For this review, take the finished solid that the model builds, in its own axes (mm). A direction names the side the tool comes from. Give positions to 0.01 mm unless a question says otherwise; leave off trailing zeros. Loops run counter-clockwise (first coordinate to the right, second up) from the corner with the lowest first, then second, coordinate; pieces in that order, holes last. Notation, with made-up numbers: (28, -9.5) - (85, -9.5) arc R13 cw to (85, -0.5) - close; hole circle Ø7 at (88.25, -26). An arc over 180 degrees is marked (long way). Answer in a Markdown table with one row per item.
```python
from build123d import *

# Parameters (mm, degrees)
SKETCH1_R                     = 44.45
SKETCH1_R_2                   = 3.25
BOSS_EXTRUDE1_DEPTH           = 3.175
BOSS_EXTRUDE2_DEPTH           = 67.31
CBORE_FOR_M6_SHCS2_AT_2_COUNT = 2
CBORE_FOR_M6_SHCS2_AT_2_PITCH = 111.76
CBORE_FOR_M6_SHCS2_AT_3_COUNT = 2
CBORE_FOR_M6_SHCS2_AT_3_PITCH = 158.052507731
CBORE_FOR_M6_SHCS2_AT_4_COUNT = 2
CBORE_FOR_M6_SHCS2_AT_4_PITCH = 111.76


with BuildPart() as part:
    # Sketch1 → Boss-Extrude1 (new body)
    with BuildSketch(Plane(origin=(0, 0, 0), x_dir=(1, 0, 0), z_dir=(0, 1, 0))):
        with BuildLine():
            Line((-57.15, 63.5), (57.15, 63.5))
            ThreePointArc((57.15, 63.5), (61.640128061, 61.640128061), (63.5, 57.15))
            Line((63.5, 57.15), (63.5, -57.15))
            ThreePointArc((63.5, -57.15), (61.640128061, -61.640128061), (57.15, -63.5))
            Line((57.15, -63.5), (-57.15, -63.5))
            ThreePointArc((-57.15, -63.5), (-61.640128061, -61.640128061), (-63.5, -57.15))
            Line((-63.5, -57.15), (-63.5, 57.15))
            ThreePointArc((-63.5, 57.15), (-61.640128061, 61.640128061), (-57.15, 63.5))
        make_face()
        Circle(SKETCH1_R, mode=Mode.SUBTRACT)
        with Locations((-57.15, 53.975)):
            Circle(SKETCH1_R_2, mode=Mode.SUBTRACT)
        with Locations((57.15, 53.975)):
            Circle(SKETCH1_R_2, mode=Mode.SUBTRACT)
        with Locations((57.15, -53.975)):
            Circle(SKETCH1_R_2, mode=Mode.SUBTRACT)
        with Locations((-57.15, -53.975)):
            Circle(SKETCH1_R_2, mode=Mode.SUBTRACT)
    extrude(amount=BOSS_EXTRUDE1_DEPTH)

    # Sketch3 → Boss-Extrude2 (add)
    with BuildSketch(Plane(origin=(0, 3.175, 0), x_dir=(1, 0, 0), z_dir=(0, 1, 0))):
        with BuildLine():
            Line((-57.15, -63.5), (57.15, -63.5))
            ThreePointArc((57.15, -63.5), (61.640128061, -61.640128061), (63.5, -57.15))
            Line((63.5, -57.15), (63.5, 57.15))
            ThreePointArc((63.5, 57.15), (61.640128061, 61.640128061), (57.15, 63.5))
            Line((57.15, 63.5), (-57.15, 63.5))
            ThreePointArc((-57.15, 63.5), (-61.640128061, 61.640128061), (-63.5, 57.15))
            Line((-63.5, 57.15), (-63.5, -57.15))
            ThreePointArc((-63.5, -57.15), (-61.640128061, -61.640128061), (-57.15, -63.5))
        make_face()
        with BuildLine():
            Line((-54.700256121, 45.358975516), (-45.358975516, 54.700256121))
            ThreePointArc((-45.358975516, 54.700256121), (-41.238798986, 57.453270063), (-36.378719395, 58.42))
            Line((-36.378719395, 58.42), (36.378719395, 58.42))
            ThreePointArc((36.378719395, 58.42), (41.238798986, 57.453270063), (45.358975516, 54.700256121))
            Line((45.358975516, 54.700256121), (54.700256121, 45.358975516))
            ThreePointArc((54.700256121, 45.358975516), (57.453270063, 41.238798986), (58.42, 36.378719395))
            Line((58.42, 36.378719395), (58.42, -36.378719395))
            ThreePointArc((58.42, -36.378719395), (57.453270063, -41.238798986), (54.700256121, -45.358975516))
            Line((54.700256121, -45.358975516), (45.358975516, -54.700256121))
            ThreePointArc((45.358975516, -54.700256121), (41.238798986, -57.453270063), (36.378719395, -58.42))
            Line((36.378719395, -58.42), (-36.378719395, -58.42))
            ThreePointArc((-36.378719395, -58.42), (-41.238798986, -57.453270063), (-45.358975516, -54.700256121))
            Line((-45.358975516, -54.700256121), (-54.700256121, -45.358975516))
            ThreePointArc((-54.700256121, -45.358975516), (-57.453270063, -41.238798986), (-58.42, -36.378719395))
            Line((-58.42, -36.378719395), (-58.42, 36.378719395))
            ThreePointArc((-58.42, 36.378719395), (-57.453270063, 41.238798986), (-54.700256121, 45.358975516))
        make_face(mode=Mode.SUBTRACT)
    extrude(amount=BOSS_EXTRUDE2_DEPTH)

    # Sketch9 → CBORE for M6 SHCS2 (revolve, cut)
    with BuildSketch(Plane(origin=(55.88, 0, -55.88), x_dir=(0, 0, -1), z_dir=(1, 0, 0))):
        Polygon((0, 0), (0, 70.485), (3.5, 70.485), (3.5, 31.4), (5.5, 31.4), (5.5, 0.025), (5.525, 0), align=None)
    cbore_for_m6_shcs2 = revolve(axis=Axis((55.88, -6.35, -55.88), (0, 1, 0)), mode=Mode.SUBTRACT)

    # CBORE for M6 SHCS2 at 2: CBORE for M6 SHCS2 ×2
    with Locations(*[(-i * CBORE_FOR_M6_SHCS2_AT_2_PITCH, 0, 0) for i in range(1, CBORE_FOR_M6_SHCS2_AT_2_COUNT)]):
        add(cbore_for_m6_shcs2, mode=Mode.SUBTRACT)

    # CBORE for M6 SHCS2 at 3: CBORE for M6 SHCS2 ×2
    with Locations(*[Vector(-0.707106781, 0, 0.707106781) * (i * CBORE_FOR_M6_SHCS2_AT_3_PITCH) for i in range(1, CBORE_FOR_M6_SHCS2_AT_3_COUNT)]):
        add(cbore_for_m6_shcs2, mode=Mode.SUBTRACT)

    # CBORE for M6 SHCS2 at 4: CBORE for M6 SHCS2 ×2
    with Locations(*[(0, 0, i * CBORE_FOR_M6_SHCS2_AT_4_PITCH) for i in range(1, CBORE_FOR_M6_SHCS2_AT_4_COUNT)]):
        add(cbore_for_m6_shcs2, mode=Mode.SUBTRACT)


solid = part.part
```
1. Clearance check with flat-ended pins moving along their axes: pin 1 (10 mm diameter, centred on x = -22.5, z = 27.5, fed in from +Y); pin 2 (12 mm diameter, centred on x = 55, z = -56.5, fed in from -Y); pin 3 (6 mm diameter, centred on x = -38, z = -22.5, fed in from +Y) (3 decimals). State where each tip first meets the part, or that it passes through.
Values:
| item | result |
|---|---|
| pin 1 | passes through |
| pin 2 | stops at y = 0 |
| pin 3 | stops at y = 3.175 |
2. We need section C-C, the plane z = 0. Give the boundary of the cut face in (x, y) (3 decimals).
Values:
| item | result |
|---|---|
| outline | (-63.5, 0) - (-44.45, 0) - (-44.45, 3.175) - (-58.42, 3.175) - (-58.42, 70.485) - (-63.5, 70.485) - close; (44.45, 0) - (63.5, 0) - (63.5, 70.485) - (58.42, 70.485) - (58.42, 3.175) - (44.45, 3.175) - close |
3. We need section B-B, the plane x = 0. Give the boundary of the cut face in (y, z) (3 decimals), and give its area (3 significant figures).
Values:
| item | result |
|---|---|
| outline | (0, -63.5) - (70.485, -63.5) - (70.485, -58.42) - (3.175, -58.42) - (3.175, -44.45) - (0, -44.45) - close; (0, 44.45) - (3.175, 44.45) - (3.175, 58.42) - (70.485, 58.42) - (70.485, 63.5) - (0, 63.5) - close |
| area | 805 mm^2 |
4. Mouldability with a two-part tool opening along X and no side actions: class faces 1 (the face through (57, 31.4, 59.5)), 2 (the face through (1, 35, -63.5)), 3 (the face through (-63.5, 35, -1)) as released by +X, released by -X, zero draft, split by the parting line, or undercut.
Values:
| item | result |
|---|---|
| face 1 | undercut |
| face 2 | zero draft |
| face 3 | released by -X |
5. For faces 4 (the face through (-50.1, 36.36, -49.96)), 5 (the face through (56, 31.4, -52)), 6 (the face through (-56.034, 50.669, -52.383)), list the 3-axis set-ups (+Z, -Z, +X, -X, +Y, -Y) from which the entire face can be reached by the end or side of a thin tool; tool diameter is ignored.
Values:
| item | result |
|---|---|
| face 4 | +Y |
| face 5 | -Y |
| face 6 | +Y, -Y |
6. We need section A-A, the plane y = 21. Give the boundary of the cut face in (x, z), and give its area (3 significant figures).
Values:
| item | result |
|---|---|
| outline | (-63.5, -57.15) arc R6.35 ccw to (-57.15, -63.5) - (57.15, -63.5) arc R6.35 ccw to (63.5, -57.15) - (63.5, 57.15) arc R6.35 ccw to (57.15, 63.5) - (-57.15, 63.5) arc R6.35 ccw to (-63.5, 57.15) - close; hole circle Ø11 at (-55.88, -55.88); hole circle Ø11 at (-55.88, 55.88); hole (-58.42, -36.38) arc R12.7 ccw to (-54.7, -45.36) - (-45.36, -54.7) arc R12.7 ccw to (-36.38, -58.42) - (36.38, -58.42) arc R12.7 ccw to (45.36, -54.7) - (54.7, -45.36) arc R12.7 ccw to (58.42, -36.38) - (58.42, 36.38) arc R12.7 ccw to (54.7, 45.36) - (45.36, 54.7) arc R12.7 ccw to (36.38, 58.42) - (-36.38, 58.42) arc R12.7 ccw to (-45.36, 54.7) - (-54.7, 45.36) arc R12.7 ccw to (-58.42, 36.38) - close; hole circle Ø11 at (55.88, -55.88); hole circle Ø11 at (55.88, 55.88) |
| area | 2,650 mm^2 |
7. We need section D-D, the plane y = 62. Give the boundary of the cut face in (x, z), and give its area (3 significant figures).
Values:
| item | result |
|---|---|
| outline | (-63.5, -57.15) arc R6.35 ccw to (-57.15, -63.5) - (57.15, -63.5) arc R6.35 ccw to (63.5, -57.15) - (63.5, 57.15) arc R6.35 ccw to (57.15, 63.5) - (-57.15, 63.5) arc R6.35 ccw to (-63.5, 57.15) - close; hole circle Ø7 at (-55.88, -55.88); hole circle Ø7 at (-55.88, 55.88); hole (-58.42, -36.38) arc R12.7 ccw to (-54.7, -45.36) - (-45.36, -54.7) arc R12.7 ccw to (-36.38, -58.42) - (36.38, -58.42) arc R12.7 ccw to (45.36, -54.7) - (54.7, -45.36) arc R12.7 ccw to (58.42, -36.38) - (58.42, 36.38) arc R12.7 ccw to (54.7, 45.36) - (45.36, 54.7) arc R12.7 ccw to (36.38, 58.42) - (-36.38, 58.42) arc R12.7 ccw to (-45.36, 54.7) - (-54.7, 45.36) arc R12.7 ccw to (-58.42, 36.38) - close; hole circle Ø7 at (55.88, -55.88); hole circle Ø7 at (55.88, 55.88) |
| area | 2,880 mm^2 |
8. Wall thickness on line 1 (X direction, y = 51.5, z = 34); line 2 (X direction, y = 8, z = -55): over which ranges is each line inside the solid? List them lowest first. Write a range as [from, to].
Values:
| item | result |
|---|---|
| line 1 | x = [-63.5, -58.42], [58.42, 63.5] |
| line 2 | x = [-63.5, -61.31], [-50.45, -45.05], [45.05, 50.45], [61.31, 63.5] |
